Job drawing, mm, ordinate dimensions from the low corner. One solid piece. Round coordinates to 2 decimals unless told otherwise and drop trailing zeros. Loops run counter-clockwise (first coordinate to the right, second up) from the corner with the lowest first, then second, coordinate; pieces in that order, holes last.
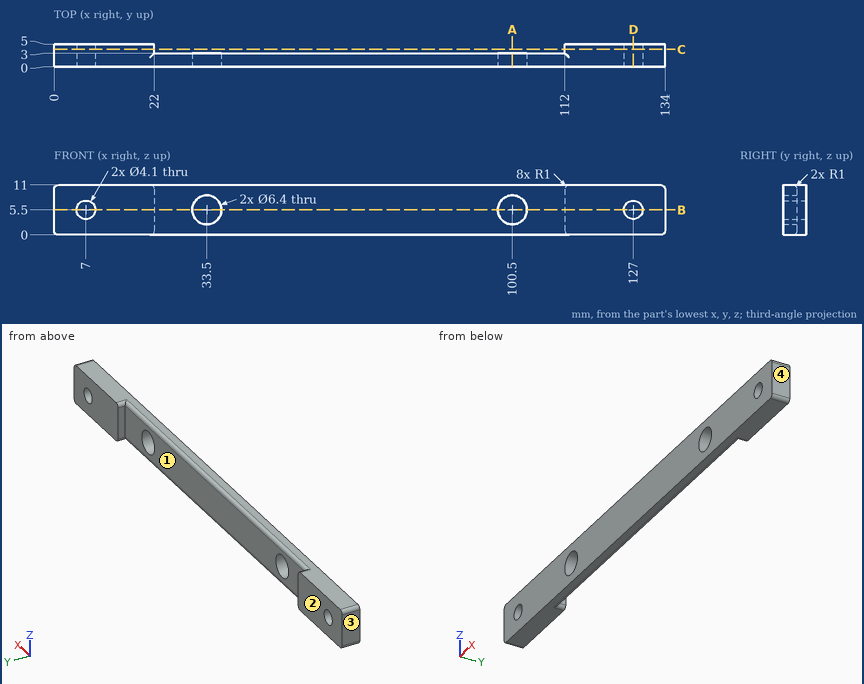
Item 1: Cut at D-D, the plane x = 127. Give the cut face in (y, z), plus the area to 3 significant figures.
Answers follow:
outline: (0, 0) - (5, 0) - (5, 3.45) - (0, 3.45) - close; (0, 7.55) - (5, 7.55) - (5, 11) - (0, 11) - close
area: 34.5 mm2
Item 2: Cut at A-A, the plane x = 100.5. Give the cut face in (y, z), plus the area to 3 significant figures.
Answers follow:
outline: (0, 0) - (2, 0) arc R1 ccw to (3, 1) - (3, 2.3) - (0, 2.3) - close; (0, 8.7) - (3, 8.7) - (3, 10) arc R1 ccw to (2, 11) - (0, 11) - close
area: 13.4 mm2
Item 3: Cut at C-C, the plane y = 3.8. Give the cut face in (x, z).
Answers follow:
outline: (0, 1) arc R1 ccw to (1, 0) - (21, 0) arc R1 ccw to (22, 1) - (22, 10) arc R1 ccw to (21, 11) - (1, 11) arc R1 ccw to (0, 10) - close; (112, 1) arc R1 ccw to (113, 0) - (133, 0) arc R1 ccw to (134, 1) - (134, 10) arc R1 ccw to (133, 11) - (113, 11) arc R1 ccw to (112, 10) - close; hole circle Ø4.1 at (7, 5.5); hole circle Ø4.1 at (127, 5.5)
Item 4: Flat gauge pins, fed straight in: P1, Ø4, axis at x = 66.5, z = 3.5, coming from the -Y side; P2, Ø6, axis at x = 100.5, z = 5.5, coming from the +Y side; P3, Ø2, axis at x = 103, z = 3.5, coming from the +Y side. Where does each tip first touch, or does it go through?
Answers follow:
P1: stops at y = 0
P2: passes through
P3: stops at y = 3
Item 5: Two-plate mould, pull along X, no slides. Class the marked faces 1, 2, 3 and 4: released by +X, released by -X, zero draft, split by the parting line, or undercut.
Answers follow:
face 1: undercut
face 2: zero draft
face 3: released by -X
face 4: released by +X
Item 6: Cut at B-B, the plane z = 5.5. Give the cut face in (x, y), plus the area to 3 significant figures.
Answers follow:
outline: (0, 0) - (4.95, 0) - (4.95, 5) - (0, 5) - close; (9.05, 0) - (30.3, 0) - (30.3, 3) - (22, 3) - (22, 5) - (9.05, 5) - close; (36.7, 0) - (97.3, 0) - (97.3, 3) - (36.7, 3) - close; (103.7, 0) - (124.95, 0) - (124.95, 5) - (112, 5) - (112, 3) - (103.7, 3) - close; (129.05, 0) - (134, 0) - (134, 5) - (129.05, 5) - close
area: 411 mm2
Item 7: Probe line 1 (X direction, y = 1.95, z = 5.5); line 2 (X direction, y = 4.5, z = 6.5); line 3 (Z direction, x = 33.5, y = 2.1). List the from-to ranges inside material, lowest first.
Answers follow:
line 1: x = 0 to 4.95, 9.05 to 30.3, 36.7 to 97.3, 103.7 to 124.95, 129.05 to 134
line 2: x = 0 to 5.21, 8.79 to 22, 112 to 125.21, 128.79 to 134
line 3: z = 0.01 to 2.3, 8.7 to 10.99
